```python
from build123d import *

# Parameters (mm, degrees)
F1_DEPTH = 44.45
F3_DEPTH = 50.8
F5_DEPTH = 95.25


with BuildPart() as f1:
    # F0 (on Front) → F1 (new body)
    with BuildSketch(Plane.XZ):
        with BuildLine():
            Line((-32.0718213916, -23.4942715615), (18.7281786084, -23.4942715615))
            Line((18.7281786084, -23.4942715615), (18.7281786084, 37.4657284385))
            ThreePointArc((18.7281786084, 37.4657284385), (-6.6718213916, 43.0537284385), (-32.0718213916, 37.4657284385))
            Line((-32.0718213916, 37.4657284385), (-32.0718213916, -23.4942715615))
        make_face()
    extrude(amount=F1_DEPTH)

    # F2 (on face) → F3 (cut)
    with BuildSketch(Plane(origin=(-32.0718213916, 0, 0), x_dir=(0, -1, 0), z_dir=(-1, 0, 0))):
        with BuildLine():
            Line((44.45, 10.9887497426), (44.45, 30.9227071344))
            ThreePointArc((44.45, 30.9227071344), (26.2820829109, 20.9557284385), (44.45, 10.9887497426))
        make_face()
    extrude(amount=-F3_DEPTH, mode=Mode.SUBTRACT)

    # F4 (on face) → F5 (join)
    with BuildSketch(Plane(origin=(0, 0, 0), x_dir=(-1, 0, 0), z_dir=(0, 1, 0))):
        with BuildLine():
            ThreePointArc((26.5125769861, 11.4307284385), (-0.0859693436, 30.0851608057), (-8.5655071407, -1.276726136))
            Line((-8.5655071407, -1.276726136), (21.9091499238, -1.276726136))
            ThreePointArc((21.9091499238, -1.276726136), (25.3262537588, 4.6729377033), (26.5125769861, 11.4307284385))
        make_face()
        with BuildLine():
            Line((-18.7281786084, -1.276726136), (-18.7281786084, -23.4942715615))
            Line((-18.7281786084, -23.4942715615), (32.0718213916, -23.4942715615))
            Line((32.0718213916, -23.4942715615), (32.0718213916, -1.276726136))
            Line((32.0718213916, -1.276726136), (21.9091499238, -1.276726136))
            ThreePointArc((21.9091499238, -1.276726136), (6.6718213916, -8.410027156), (-8.5655071407, -1.276726136))
            Line((-8.5655071407, -1.276726136), (-18.7281786084, -1.276726136))
        make_face()
        with BuildLine():
            Line((21.9091499238, -1.276726136), (-8.5655071407, -1.276726136))
            ThreePointArc((-8.5655071407, -1.276726136), (6.6718213916, -8.410027156), (21.9091499238, -1.276726136))
        make_face()
    extrude(amount=F5_DEPTH)


solid = f1.part
```
Input: part model. Units: mm. Frame: model coordinates. A direction names the side the tool comes from. Round coordinates to 2 decimals unless told otherwise and drop trailing zeros. Loops run counter-clockwise (first coordinate to the right, second up) from the corner with the lowest first, then second, coordinate; pieces in that order, holes last. Notation, with made-up numbers: (3.25, 46.25) - (10.25, 46.25) arc R18 cw to (10.25, 58.25) - close; hole circle Ø9 at (-11, 81.25). An arc over 180 degrees is marked (long way). One line per item, written item: value. Start each with the question number.
(1) Contact query for flat-ended pins moving along their axis: P1, Ø8, axis at x = 14, y = 39.5, coming from the +Z side; P2, Ø1, axis at x = -26.5, z = 23, coming from the -Y side; P3, Ø3, axis at x = -25, y = 69, coming from the +Z side. Output: stop coordinate, or through.
(2) Section A-A, the plane y = -38.1. Return loops of the section in (x, z).
(3) Section B-B, the plane z = 20. Return loops of the section in (x, y).
(4) Section C-C, the plane x = -10. Return loops of the section in (y, z), plus the area to 3 significant figures.
(5) Section D-D, the plane y = 5. Return loops of the section in (x, z), plus the area to 3 significant figures.
(6) Draft query along Y for faces 1 (the cylindrical face through (-7.027, -26.287, 21.309)), 2 (the flat face through (14, 47, -1.277)), 3 (the flat face through (-6, 95.25, -2)). Return one class per face: +Y half, -Y half, draft (parallel to the pull), parting line (faces both ways), or undercut.
(7) Ray query, line 1 (Z direction, x = -7, y = -38.1); line 2 (Z direction, x = 1.5, y = -38.1); line 3 (Y direction, x = 14, z = 6). Return the intervals inside material, ascending. Write a range as [from, to].
(8) Access query for faces 4 (the flat face through (-27, 47, -1.277)), 5 (the flat face through (-7, -44.45, 36)). Directions: +Z, -Z, +X, -X, +Y, -Y. A direction counts if a zero-diameter tool reaches every point of the face in a straight line with its end or side. Return the directions, or none.
Results below:
1. P1: z = 22.19
1. P2: y = -26.56
1. P3: z = 21.94
2. outline: (-32.07, -23.49) - (18.73, -23.49) - (18.73, 9.14) - (-32.07, 9.14) - close; (-32.07, 32.77) - (18.73, 32.77) - (18.73, 37.47) arc R60.52 ccw to (-32.07, 37.47) - close
3. outline: (-32.07, -26.32) - (18.73, -26.32) - (18.73, 0) - (11.22, 0) - (11.22, 95.25) - (-24.57, 95.25) - (-24.57, 0) - (-32.07, 0) - close
4. outline: (-44.45, -23.49) - (95.25, -23.49) - (95.25, 30.99) - (0, 30.99) - (0, 42.96) - (-44.45, 42.96) - (-44.45, 30.92) arc R11.82 cw (long way) to (-44.45, 10.99) - close
4. area: 7,780 mm^2
5. outline: (-32.07, -23.49) - (18.73, -23.49) - (18.73, -1.28) - (8.57, -1.28) arc R19.84 ccw (long way) to (-21.91, -1.28) - (-32.07, -1.28) - close
5. area: 2,210 mm^2
6. face 1: undercut
6. face 2: draft
6. face 3: +Y half
7. line 1: [-23.49, 9.14], [32.77, 43.05]
7. line 2: [-23.49, 9.14], [32.77, 42.5]
7. line 3: [-44.45, 0]
8. face 4: -X, +Y
8. face 5: +Z, -Z, +X, -X, -Y
